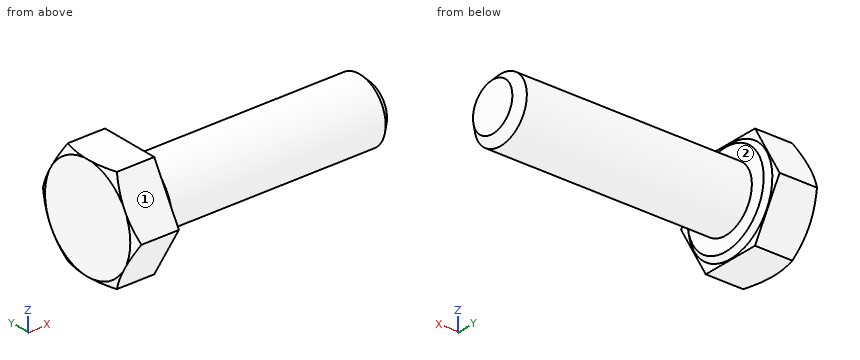
from build123d import *

# Parameters (mm, degrees)
EXTRUDE_1_DEPTH = 2.65
CHAMFER_2_SIZE  = 1


with BuildPart() as part:
    # 草图1 → 拉伸1 (new, symmetric)
    with BuildSketch(Plane(origin=(0, 0, 0), x_dir=(0, 0, 1), z_dir=(1, 0, 0))):
        Polygon((0, 7.505553499), (-6.5, 3.75277675), (-6.5, -3.75277675), (0, -7.505553499), (6.5, -3.75277675), (6.5, 3.75277675), align=None)
    extrude(amount=EXTRUDE_1_DEPTH, both=True)

    # 草图2 → 切除-旋转2 (revolve, cut)
    with BuildSketch(Plane.XY):
        Polygon((-2.65, 6.5), (0.034663773, 11.149974056), (-2.65, 11.149974056), align=None)
    revolve(axis=Axis((-3.243026821, 0, 0), (1, 0, 0)), mode=Mode.SUBTRACT)

    # 草图3 → 旋转1 (revolve)
    with BuildSketch(Plane.XY, mode=Mode.PRIVATE) as revolve_1_sk:
        Polygon((2.65, 0), (2.65, 6.4), (3.25, 5.8), (3.25, 4), (32.65, 4), (32.65, 0), align=None)
    revolve(revolve_1_sk.sketch.rotate(Axis((-4.543756915, 0, 0), (1, 0, 0)), 90), axis=Axis((-4.543756915, 0, 0), (1, 0, 0)))

    # 倒角2
    chamfer_2_edges = [part.edges().sort_by_distance(p)[0] for p in [
        (32.65, 0, -4),
    ]]
    chamfer(chamfer_2_edges, length=CHAMFER_2_SIZE)


solid = part.part
Work out the finished part from the listing and answer in its coordinate system (mm). Face numbers are marked on the shaded views. A direction names the side the tool comes from. Round coordinates to 2 decimals unless told otherwise and drop trailing zeros. Loops run counter-clockwise (first coordinate to the right, second up) from the corner with the lowest first, then second, coordinate; pieces in that order, holes last. Notation, with made-up numbers: (-34, 66.5) -> (-7, 66.5) arc R23 cw to (-7, 92.5) -> close; hole circle Ø10 at (-26, 88). An arc over 180 degrees is marked (long way). Use one line per item in the form item = value.
(1) Straight lines are drawn through the part: line 1 (Y direction, x = 7, z = -3); line 2 (X direction, y = -4.25, z = -1); line 3 (Y direction, x = 16, z = -0.5). For each, find the intervals that lie inside material, in ascending order.
Answer list:
line_1 = -2.65 to 2.65
line_2 = -2.65 to 3.25
line_3 = -3.97 to 3.97
(2) A tool of negligible diameter and unlimited length cuts with its end or side. For the marked faces 1 and 2, from which of +Z, -Z, +X, -X, +Y, -Y can it reach the whole face along a straight path? Write none if from no direction.
Answer list:
face_1 = +Z, +X, -X, -Y
face_2 = +X
(3) Flat-ended cylindrical pins translate along their axes: P1, Ø5, axis at x = 12, y = -4.5, coming from the +Z side; P2, Ø2, axis at x = 25, z = 1, coming from the -Y side; P3, Ø3, axis at x = 7.5, z = -2, coming from the +Y side. Find the tip coordinate at first contact, or state that the pin passes through.
Answer list:
P1 = 3.46
P2 = -4
P3 = 3.97
(4) Find section A-A on x = 6.5. Give the vertices of the cut face in (y, z).
Answer list:
outline = circle Ø8 at (0, 0)
